Autodesk Inventor part; units mm, degrees
ref_plane "YZ Plane" through (0, 0, 0) normal (1, 0, 0) x (0, 1, 0)
ref_plane "XZ Plane" through (0, 0, 0) normal (0, 1, 0) x (-1, 0, 0)
ref_plane "XY Plane" through (0, 0, 0) normal (0, 0, 1) x (1, 0, 0)
sketch "Sketch4" plane through (0, 0, 0) normal (0, 0, 1) x (1, 0, 0)
  line L0 (-2.1, 0) -> (3, 0)
  line L1 (0, 0) -> (-2.1, 0)
  line L2 (0, 2.5) -> (0, 1.725)
  line L3 (0.5, 1.225) -> (0.5, 1.225)
  line L4 (0.5, 1.225) -> (0.9, 1.25)
  arc A0 (0, 1.725) -> (0.5, 1.225) centre (0.5, 1.725) ccw
  line L5 (-2.1, 0) -> (-2.1, 1.25)
  line L6 (0, 2.5) -> (-1.1375, 2.5)
  arc A1 (-1.1375, 2.5) -> (-2.1, 1.25) centre (1.4883, -0.5175) ccw
  line L7 (0.9, 1.25) -> (3, 1.25)
  line L8 (3, 1.25) -> (3, 0)
  point P0 (0, 1.225)
  dimension "d71" = 0.5
  dimension "d72" = 3
  dimension "d74" = 0.4
  dimension "d75" = 2.45
  dimension "d78" = 2.5
  dimension "d82" = 4
  dimension "d83" = 2.1
  dimension "d84" = 5
  dimension "d104" = 2.1
  dimension "d105" = 2.5
revolve "Revolution7" add sketch "Sketch4" angle 360 about axis through (-2.1, 0, 0) along (1, 0, 0)
sketch "Sketch5" plane through (-2.1, 0, 0) normal (-1, 0, 0) x (0, 0, 1)
  circle A0 centre (0, 0) radius 1.2 construction
  circle A1 centre (0, 0) radius 0.84 construction
  line L0 (0, 0) -> (-0.7275, 0.42)
  line L1 (0, 0) -> (-0.7275, -0.42)
  line L2 (-1.8008, 0) -> (1.7887, 0)
  line L3 (-1.2, 0) -> (-0.7275, -0.42)
  line L4 (-1.2, 0) -> (-0.7275, 0.42)
  dimension "d88" = 2.4
  dimension "d89" = 1.68
  dimension "d90" = 30
  dimension "d91" = 30
extrude "Extrusion1" cut sketch "Sketch5" against normal blind 1.04
pattern_circular "Circular Pattern1" count 6 over 360 about axis through (-10, 0, 0) along (1, 0, 0) of "Extrusion1"
fillet "Fillet1" radius 0.24 12 edges at (-1.58, -1.0392, -0.6) (-1.58, -0.42, -0.7275) (-1.58, -0.84, 0) (-1.58, -1.0392, 0.6) (-1.58, -0.42, 0.7275) (-1.58, 0, 1.2) (-1.58, 0.84, 0) (-1.58, 1.0392, 0.6) (-1.58, 0.42, 0.7275) (-1.58, 0.42, -0.7275) (-1.58, 0, -1.2) (-1.58, 1.0392, -0.6)
thread "Thread7"
properties part number "Flachkopfschraube mit Innenrund ISO 14583 - M2,5 x 3 - 4.8" material "Stahl"
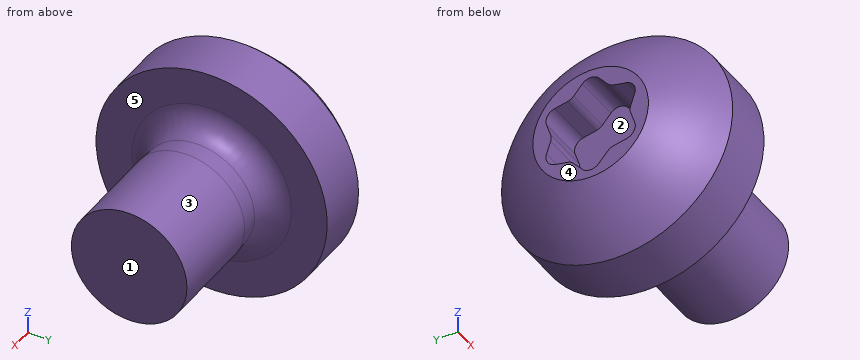
Here's how the part is built. I have some questions about the finished solid (model axes, mm). Face numbers are marked on the shaded views. A direction names the side the tool comes from. Give positions to 0.01 mm unless a question says otherwise; leave off trailing zeros. Order: outer loops, then holes, each group sorted by start corner. A loop starts at its lowest first (then second) coordinate and runs counter-clockwise, first axis right, second up. Notation, with made-up numbers: (26.25, 1) - (79.25, 1) arc R17 cw to (79.25, 24) - close; hole circle Ø10 at (-20, 28). An arc over 180 degrees is marked (long way). Answer as a JSON object with one key per item and string values. Group by question number.
Item 1: If we section it at A-A on x = 2.15: Please give me the cut outline in (y, z), and give its area (3 significant figures).
Item 2: For P1, Ø3, axis at x = -0.5, z = 0.5, coming from the -Y side; P2, Ø1.5, axis at x = 2.5, y = 0.5, coming from the -Z side, each with a flat end and sliding along its axis, tell me the tip position at first contact or that it passes through.
Item 3: If we section it at B-B on x = 0.3: Please give me the cut outline in (y, z).
Item 4: If we mould it in two halves opening along Z, with no side actions, what happens to the marked faces 1, 2 and 3? For each: pulls with the +Z half, pulls with the -Z half, needs draft (parallel to the pull), parting line crosses it, or undercut.
Item 5: Please list where these lines run through material, in increasing order: probe 1 along Z at (x, y) = (2, 0.9); probe 2 along X at (y, z) = (0.15, 0.6); probe 3 along X at (y, z) = (-1.6, -1.25).
Item 6: Which directions (+Z, -Z, +X, -X, +Y, -Y) give clear straight access to the entire face, cutting with the end or side of a thin tool? Please do the marked faces 4 and 5.
Result set:
{
 "1": {"outline": "circle Ø2.5 at (0, 0)", "area": "4.91 mm²"},
 "2": {"P1": "y = -2.5", "P2": "z = -1.25"},
 "3": {"outline": "circle Ø2.53 at (0, 0)"},
 "4": {"face 1": "needs draft", "face 2": "undercut", "face 3": "parting line crosses it"},
 "5": {"probe 1": "-0.87 to 0.87", "probe 2": "-1.06 to 3", "probe 3": "-1.6 to 0"},
 "6": {"face 4": "+Z, -Z, -X, +Y, -Y", "face 5": "+X"}
}
